Autodesk Inventor part; units mm, degrees
ref_plane "YZ Plane" through (0, 0, 0) normal (1, 0, 0) x (0, 1, 0)
ref_plane "XZ Plane" through (0, 0, 0) normal (0, 1, 0) x (-1, 0, 0)
ref_plane "XY Plane" through (0, 0, 0) normal (0, 0, 1) x (1, 0, 0)
sketch "Pole Base Profile" plane through (0, 0, 0) normal (0, 1, 0) x (-1, 0, 0)
  line L0 (3.5, 2.75) -> (-3.5, 2.75)
  line L1 (-3.5, 2.75) -> (-3.5, -2.75)
  line L2 (-3.5, -2.75) -> (3.5, -2.75)
  line L3 (3.5, -2.75) -> (3.5, 2.75)
  line L4 (3.5, 2.75) -> (-3.5, -2.75) construction
  line L5 (-3.5, 2.75) -> (3.5, -2.75) construction
  point P0 (0, 0)
  dimension "d0" = 7
  dimension "d1" = 5.5
extrude "Pole Base" add sketch "Pole Base Profile" along normal blind 3
sketch "Cross Base" plane through (0, 3, 0) normal (0, 1, 0) x (1, 0, 0)
  line L0 (-0.8, -2.175) -> (0.8, -2.175)
  line L1 (0.8, -2.175) -> (0.8, 2.175)
  line L2 (0.8, 2.175) -> (-0.8, 2.175)
  line L3 (-0.8, 2.175) -> (-0.8, -2.175)
  line L4 (-0.8, -2.175) -> (0.8, 2.175) construction
  line L5 (0.8, -2.175) -> (-0.8, 2.175) construction
  line L6 (-2.175, -0.8) -> (2.175, -0.8)
  line L7 (2.175, -0.8) -> (2.175, 0.8)
  line L8 (2.175, 0.8) -> (-2.175, 0.8)
  line L9 (-2.175, 0.8) -> (-2.175, -0.8)
  line L10 (-2.175, -0.8) -> (2.175, 0.8) construction
  line L11 (2.175, -0.8) -> (-2.175, 0.8) construction
  point P0 (0, 0)
  dimension "d12" = 1.6
  dimension "d13" = 4.35
  dimension "d14" = 4.35
  dimension "d15" = 1.6
extrude "Pole" add sketch "Cross Base" along normal blind 3.6
fillet "Pole Rounding" radius 0.25 8 edges at (2.175, 4.8, 0.8) (0.8, 4.8, 2.175) (-0.8, 4.8, 2.175) (-2.175, 4.8, 0.8) (-2.175, 4.8, -0.8) (-0.8, 4.8, -2.175) (0.8, 4.8, -2.175) (2.175, 4.8, -0.8)
fillet "Base Rounding" radius 0.3 4 edges at (-3.5, 3, 0) (0, 3, -2.75) (0, 3, 2.75) (3.5, 3, 0)
sketch "Top Center Point" plane through (0, 6.6, 0) normal (0, 1, 0) x (1, 0, 0)
  point P0 (0, 0)
equation "\"d0\" = s_polebl"
equation "\"d1\" = s_polebw"
equation "\"d12\" = k_cmxw"
equation "\"d13\" = k_cmxl"
equation "\"d14\" = d13"
equation "\"d15\" = d12"
equation "\"d8\" = s_poleh"
equation "\"k_width\" = 18.1"
equation "\"k_height\" = 18"
equation "\"k_taper1\" = 1.5"
equation "\"k_taper2\" = 0.5"
equation "\"k_radius\" = 6"
equation "\"k_wthick\" = 1.5"
equation "\"k_ribthick\" = 1.5"
equation "\"k_ribheight\" = 5"
equation "\"k_poleoff\" = 2.2625"
equation "\"k_poledia\" = 5.54"
equation "\"k_cmxw\" = 1.6"
equation "\"k_cmxl\" = 4.35"
equation "\"s_bwidth\" = 15.6"
equation "\"s_poleh\" = 3.6"
equation "\"s_polebw\" = 5.5"
equation "\"s_polebl\" = 7"
equation "\"b_rshift\" = 49.775"
equation "\"b_height\" = 77.4"
equation "\"b_tab\" = 27.15"
equation "\"b_lshift\" = 40.725"
equation "\"b_space\" = 117.65"
equation "\"b_caps\" = 31.675"
equation "\"b_pad\" = 1"
equation "\"b_width\" = 286.5"
equation "\"b_ctrl\" = 22.625"
equation "\"k_staper\" = 1"
equation "\"k_ltaper\" = 1.5"
equation "\"k_sradius\" = 4"
equation "\"k_lradius\" = 6"
equation "\"k_height_t\" = 16"
equation "\"k_height_low\" = 16"
equation "\"k_taper_wide\" = 1.5"
equation "\"k_taper_thin\" = 0.5"
properties part number "keyswitch-pole_cherrymx"
Input: part model. Units: mm. Frame: model coordinates. A direction names the side the tool comes from. Round coordinates to 2 decimals unless told otherwise and drop trailing zeros. Loops run counter-clockwise (first coordinate to the right, second up) from the corner with the lowest first, then second, coordinate; pieces in that order, holes last. Notation, with made-up numbers: M -34,21 L 12,21 A15 cw 12,40 Z; hole C 84,12 d8. An arc over 180 degrees is marked long. Answer as CSV lines item,"result". Start each with the question number.
(1) First-contact query: pin 1 (0.6 mm diameter, centred on x = 0, y = 4.5, fed in from +Z) (3 decimals); pin 2 (1.2 mm diameter, centred on y = 5, z = 0, fed in from -X) (3 decimals); pin 3 (1.2 mm diameter, centred on x = -1.5, y = 4.5, fed in from +Z). Flat tips, straight axial feed; report the tip coordinate or a pass-through.
(2) Section B-B, the plane x = -1. Output: boundary loops of the cut face in (y, z).
(3) Line query: line 1 (Z direction, x = -1.75, y = 5); line 2 (Y direction, x = -1.75, z = -2.4); line 3 (Z direction, x = 0.5, y = 6.25) (3 decimals). Output: solid intervals per line, ascending. Write a range as [from, to].
(4) Reachability of faces 1 (the flat face through (1, 5, -0.8)), 2 (the flat face through (-1, 5, 0.8)), 3 (the flat face through (2.175, 5, 0)), 4 (the flat face through (1, 5, 0.8)), 5 (the flat face through (0, 5, 2.175)) from +Z, -Z, +X, -X, +Y, -Y: full face, straight path, thin tool, end or side. Return the list, or none.
(5) Section A-A, the plane z = -1.8. Output: boundary loops of the cut face in (x, y), plus the area to 3 significant figures.
(6) Section D-D, the plane x = 3. Output: boundary loops of the cut face in (y, z).
(7) Section C-C, the plane y = 5.25. Output: boundary loops of the cut face in (x, z) (3 decimals).
Values found:
1,pin 1,"stops at z = 2.175"
1,pin 2,"stops at x = -2.175"
1,pin 3,"stops at z = 0.8"
2,outline,"M 0,-2.75 L 2.7,-2.75 A0.3 ccw 3,-2.45 L 3,-0.8 L 6.6,-0.8 L 6.6,0.8 L 3,0.8 L 3,2.45 A0.3 ccw 2.7,2.75 L 0,2.75 Z"
3,line 1,"z = [-0.8, 0.8]"
3,line 2,"y = [0, 3]"
3,line 3,"z = [-2.175, 2.175]"
4,face 1,"-Z, +X, +Y"
4,face 2,"+Z, -X, +Y"
4,face 3,"+Z, -Z, +X, +Y"
4,face 4,"+Z, +X, +Y"
4,face 5,"+Z, +X, -X, +Y"
5,outline,"M -3.5,0 L 3.5,0 L 3.5,2.7 A0.3 ccw 3.2,3 L 0.8,3 L 0.8,6.6 L -0.8,6.6 L -0.8,3 L -3.2,3 A0.3 ccw -3.5,2.7 Z"
5,area,"26.7 mm²"
6,outline,"M 0,-2.75 L 2.7,-2.75 A0.3 ccw 3,-2.45 L 3,2.45 A0.3 ccw 2.7,2.75 L 0,2.75 Z"
7,outline,"M -2.175,-0.55 A0.25 ccw -1.925,-0.8 L -0.8,-0.8 L -0.8,-1.925 A0.25 ccw -0.55,-2.175 L 0.55,-2.175 A0.25 ccw 0.8,-1.925 L 0.8,-0.8 L 1.925,-0.8 A0.25 ccw 2.175,-0.55 L 2.175,0.55 A0.25 ccw 1.925,0.8 L 0.8,0.8 L 0.8,1.925 A0.25 ccw 0.55,2.175 L -0.55,2.175 A0.25 ccw -0.8,1.925 L -0.8,0.8 L -1.925,0.8 A0.25 ccw -2.175,0.55 Z"
